Autodesk Inventor part; units mm, degrees
ref_plane "YZ Plane" through (0, 0, 0) normal (1, 0, 0) x (0, 1, 0)
ref_plane "XZ Plane" through (0, 0, 0) normal (0, 1, 0) x (-1, 0, 0)
ref_plane "XY Plane" through (0, 0, 0) normal (0, 0, 1) x (1, 0, 0)
sketch "Sketch1" plane through (0, 0, 0) normal (1, 0, 0) x (0, 1, 0)
  line L0 (0, 0) -> (33.25, 0)
  line L1 (33.25, 0) -> (33.25, -33.25)
  line L2 (33.25, -33.25) -> (0, -33.25)
  line L3 (0, -33.25) -> (0, 0)
  dimension "d0" = 33.25
  dimension "d1" = 33.25
extrude "Extrusion1" add sketch "Sketch1" along normal blind 30
sketch "Sketch2" plane through (30, 0, 0) normal (1, 0, 0) x (0, 0, -1)
  line L0 (3.25, 3.25) -> (30, 3.25)
  line L1 (30, 3.25) -> (30, 30)
  line L2 (30, 30) -> (3.25, 30)
  line L3 (3.25, 30) -> (3.25, 3.25)
  point P0 (0, 0)
  dimension "d4" = 26.75
  dimension "d5" = 26.75
sketch "Sketch3" plane through (30, 0, 0) normal (1, 0, 0) x (0, 0, -1)
  line L0 (33.25, 0) -> (33.25, 33.25)
  line L1 (0, 0) -> (33.25, 0)
  line L2 (33.25, 0) -> (33.25, 33.25)
  line L3 (33.25, 33.25) -> (0, 33.25)
  line L4 (0, 33.25) -> (0, 0)
sketch "Sketch4" plane through (30, 0, 0) normal (1, 0, 0) x (0, 0, -1)
  line L0 (3.25, 3.25) -> (30, 3.25)
  line L1 (30, 3.25) -> (30, 30)
  line L2 (30, 30) -> (3.25, 30)
  line L3 (3.25, 30) -> (3.25, 3.25)
  line L4 (0, 33.25) -> (0, 0)
  line L5 (33.25, 0) -> (33.25, 33.25)
  line L6 (0, 0) -> (33.25, 0)
  line L7 (33.25, 0) -> (33.25, 33.25)
  line L8 (33.25, 33.25) -> (0, 33.25)
  line L9 (0, 33.25) -> (0, 0)
  dimension "d6" = 26.75
  dimension "d7" = 26.75
extrude "Extrusion2" cut sketch "Sketch4" against normal blind 3
chamfer "Chamfer1" distance 1.875 angle 45 8 edges at (13.5, 33.25, 0) (13.5, 33.25, -33.25) (28.5, 30, -3.25) (28.5, 30, -30) (28.5, 3.25, -3.25) (13.5, 0, 0) (28.5, 3.25, -30) (13.5, 0, -33.25)
sketch "Sketch5" plane through (30, 0, 0) normal (1, 0, 0) x (0, 0, -1)
  line L0 (9.875, 9.875) -> (23.375, 9.875)
  line L1 (23.375, 9.875) -> (23.375, 23.375)
  line L2 (23.375, 23.375) -> (9.875, 23.375)
  line L3 (9.875, 23.375) -> (9.875, 9.875)
  line L4 (28.125, 30) -> (5.125, 30)
  line L5 (30, 5.125) -> (30, 28.125)
  line L6 (3.25, 3.25) -> (30, 3.25)
  line L7 (30, 3.25) -> (30, 30)
  line L8 (30, 30) -> (3.25, 30)
  line L9 (3.25, 30) -> (3.25, 3.25)
  point P0 (0, 0)
  dimension "d13" = 13.5
  dimension "d14" = 13.5
  dimension "d15" = 6.625
  dimension "d16" = 6.625
extrude "Extrusion3" cut sketch "Sketch5" against normal blind 26.75 contours L3 L2 L1 L0
sketch "Sketch6" plane through (0, 1.875, 0) normal (0, 0, 1) x (1, 0, 0)
  point P0 (0, -1.875)
properties part number "cuvette holder block"
For this review, take the finished solid that the model builds, in its own axes (mm). A direction names the side the tool comes from. Coordinates: 2 decimals unless noted, no trailing zeros. Write each loop counter-clockwise with the first axis right and the second up, starting at its lowest first coordinate (ties: lowest second). Pieces come first, ordered by that corner, then holes. Notation, with made-up numbers: (18, 89) - (32, 89) arc R9 ccw to (32, 95) - close; hole circle Ø4 at (11.5, 12.25). An arc over 180 degrees is marked (long way). Put each result on its own line as item: value.
1. Add section A-A, the plane x = 24.75. Give the boundary of the cut face in (y, z) (3 decimals), then the cut area to 3 significant figures.
Values found:
outline: (0, -31.375) - (1.875, -33.25) - (31.375, -33.25) - (33.25, -31.375) - (33.25, -1.875) - (31.375, 0) - (1.875, 0) - (0, -1.875) - close; hole (9.875, -23.375) - (23.375, -23.375) - (23.375, -9.875) - (9.875, -9.875) - close
area: 916 mm²
2. Mouldability with a two-part tool opening along Z and no side actions: class faces 1 (the flat face through (13.311, 32.299, -32.326)), 2 (the flat face through (28.521, 29.049, -4.174)), 3 (the flat face through (17, 9.875, -17)) as released by +Z, released by -Z, zero draft, split by the parting line, or undercut.
Values found:
face 1: released by -Z
face 2: released by +Z
face 3: undercut
3. Wall thickness on probe 1 along Z at (x, y) = (22.25, 17) (3 decimals); probe 2 along Y at (x, z) = (27.75, -22.5) (3 decimals); probe 3 along Y at (x, z) = (16.5, -16.5) (3 decimals): over which ranges is each line inside the solid? List them lowest first.
Values found:
probe 1: -33.25 to -23.375, -9.875 to 0
probe 2: 3.25 to 9.875, 23.375 to 30
probe 3: 0 to 9.875, 23.375 to 33.25
4. Add section D-D, the plane y = 24. Give the boundary of the cut face in (x, z).
Values found:
outline: (0, -33.25) - (27, -33.25) - (27, -30) - (30, -30) - (30, -3.25) - (27, -3.25) - (27, 0) - (0, 0) - close
5. For pin 1 (0.9 mm diameter, centred on x = 28, z = -22, fed in from +Y); pin 2 (1.5 mm diameter, centred on x = 29, z = -20, fed in from -Y); pin 3 (0.9 mm diameter, centred on x = 28.5, y = 13, fed in from +Z); pin 4 (8 mm diameter, centred on x = 12.5, y = 30, fed in from +Z), all flat-tipped, find the tip position at first contact; note any pin that passes through.
Values found:
pin 1: y = 30
pin 2: y = 3.25
pin 3: z = -3.25
pin 4: z = 0
6. Add section B-B, the plane y = 20. Give the boundary of the cut face in (x, z) (3 decimals).
Values found:
outline: (0, -33.25) - (27, -33.25) - (27, -30) - (30, -30) - (30, -23.375) - (3.25, -23.375) - (3.25, -9.875) - (30, -9.875) - (30, -3.25) - (27, -3.25) - (27, 0) - (0, 0) - close
7. Machinability: for faces 4 (the flat face through (17, 23.375, -17)), 5 (the flat face through (29, 16, -30)), 6 (the flat face through (29, 30, -17)), 7 (the flat face through (28.521, 29.076, -29.049)), which of the approach directions +Z, -Z, +X, -X, +Y, -Y give a long, thin tool a straight path to every point of the face, cutting with its end or side? Answer none if there is none.
Values found:
face 4: +X
face 5: -Z, +X, +Y, -Y
face 6: +Z, -Z, +X, +Y
face 7: -Z, +X, +Y
8. Add section C-C, the plane z = -7.5. Give the boundary of the cut face in (x, y).
Values found:
outline: (0, 0) - (27, 0) - (27, 3.25) - (30, 3.25) - (30, 30) - (27, 30) - (27, 33.25) - (0, 33.25) - close
